from build123d import *

# Parameters (mm, degrees)
RESSALTO_EXTRUS_O1_DEPTH = 48
ESBO_O12_R               = 1.5
CORTE_EXTRUS_O10_DEPTH   = 10
ESBO_O13_R               = 1.5
CORTE_EXTRUS_O11_DEPTH   = 10
ESBO_O14_R               = 1.5
CORTE_EXTRUS_O12_DEPTH   = 10
ESBO_O15_R               = 1.5
CORTE_EXTRUS_O13_DEPTH   = 10
CORTE_EXTRUS_O14_DEPTH   = 10
CORTE_EXTRUS_O15_DEPTH   = 24
ESBO_O17_R               = 4
ESBO_O17_W               = 2.8
ESBO_O17_H               = 2.8
RESSALTO_EXTRUS_O2_DEPTH = 4
CORTE_EXTRUS_O16_DEPTH   = 24


with BuildPart() as part:
    # Model → Ressalto-extrusão1 (new body)
    with BuildSketch(Plane.XY):
        with BuildLine():
            Line((-0.7, 0), (39, 0))
            Line((39, 0), (39.7, 0))
            Line((39.7, 0), (39.7, -11.380317396))
            Line((39.7, -11.380317396), (50.182424304, -21.8627417))
            Line((50.182424304, -21.8627417), (58.119682605, -29.8))
            Line((58.119682605, -29.8), (81.7, -29.8))
            ThreePointArc((81.7, -29.8), (105.905643752, -13.626305928), (100.226197667, 14.926197667))
            Line((100.226197667, 14.926197667), (65.00338056, 50.149014774))
            Line((65.00338056, 50.149014774), (50.111140335, 50.149014774))
            Line((50.111140335, 50.149014774), (14.181595121, 50.149014774))
            Line((14.181595121, 50.149014774), (-3.2, 32.767419653))
            Line((-3.2, 32.767419653), (-3.2, 5))
            Line((-3.2, 5), (-3.2, 0))
            Line((-3.2, 0), (-0.7, 0))
        make_face()
        with BuildLine():
            Line((-0.7, 2.5), (39, 2.5))
            Line((39, 2.5), (39.7, 2.5))
            Line((39.7, 2.5), (42.2, 2.5))
            Line((42.2, 2.5), (42.2, -10.34478349))
            Line((42.2, -10.34478349), (51.950191257, -20.094974747))
            Line((51.950191257, -20.094974747), (59.15521651, -27.3))
            Line((59.15521651, -27.3), (81.7, -27.3))
            ThreePointArc((81.7, -27.3), (103.595944921, -12.669597347), (98.458430714, 13.158430714))
            Line((98.458430714, 13.158430714), (63.967846654, 47.649014774))
            Line((63.967846654, 47.649014774), (50.111140335, 47.649014774))
            Line((50.111140335, 47.649014774), (15.217129027, 47.649014774))
            Line((15.217129027, 47.649014774), (-0.7, 31.731885747))
            Line((-0.7, 31.731885747), (-0.7, 2.5))
        make_face(mode=Mode.SUBTRACT)
    extrude(amount=RESSALTO_EXTRUS_O1_DEPTH)

    # Esboço12 → Corte-extrusão10 (cut)
    with BuildSketch(Plane(origin=(57.576197667, 57.576197667, 0), x_dir=(0, 0, -1), z_dir=(0.707106781, 0.707106781, 0))):
        with Locations((-44, -20.072657306)):
            Circle(ESBO_O12_R)
        with Locations((-44, -52.072657306)):
            Circle(ESBO_O12_R)
    extrude(amount=-CORTE_EXTRUS_O10_DEPTH, mode=Mode.SUBTRACT)

    # Esboço13 → Corte-extrusão11 (cut)
    with BuildSketch(Plane(origin=(0, 50.149014774, 0), x_dir=(1, 0, 0), z_dir=(0, 1, 0))):
        with Locations((39.59248784, -44)):
            Circle(ESBO_O13_R)
    extrude(amount=-CORTE_EXTRUS_O11_DEPTH, mode=Mode.SUBTRACT)

    # Esboço14 → Corte-extrusão12 (cut)
    with BuildSketch(Plane.ZY.offset(3.2)):
        with Locations((44, 23.701037279)):
            Circle(ESBO_O14_R)
        with Locations((44, 7.740898975)):
            Circle(ESBO_O14_R)
    extrude(amount=-CORTE_EXTRUS_O12_DEPTH, mode=Mode.SUBTRACT)

    # Esboço15 → Corte-extrusão13 (cut)
    with BuildSketch(Plane(origin=(14.159841302, 14.159841302, 0), x_dir=(0, 0, 1), z_dir=(-0.707106781, -0.707106781, 0))):
        with Locations((44, -46.881179593)):
            Circle(ESBO_O15_R)
    extrude(amount=-CORTE_EXTRUS_O13_DEPTH, mode=Mode.SUBTRACT)

    # Esboço16 → Corte-extrusão14 (cut)
    with BuildSketch(Plane.XY.offset(48)):
        Polygon((39.7, 0), (39.7, -7.84478349), (42.2, -10.34478349), (42.2, 2.5), (-0.7, 2.5), (-0.7, 0), align=None)
    extrude(amount=-CORTE_EXTRUS_O14_DEPTH, mode=Mode.SUBTRACT)

    # Esboço18 → Corte-extrusão15 (cut)
    with BuildSketch(Plane(origin=(0, 0, 0), x_dir=(-1, 0, 0), z_dir=(0, 0, -1))):
        with BuildLine():
            Line((-39.7, 0), (3.2, 0))
            Line((3.2, 0), (3.2, 32.767419653))
            Line((3.2, 32.767419653), (-14.181595121, 50.149014774))
            Line((-14.181595121, 50.149014774), (-65.00338056, 50.149014774))
            Line((-65.00338056, 50.149014774), (-100.226197667, 14.926197667))
            ThreePointArc((-100.226197667, 14.926197667), (-105.905643752, -13.626305928), (-81.7, -29.8))
            Line((-81.7, -29.8), (-58.119682605, -29.8))
            Line((-58.119682605, -29.8), (-39.7, -11.380317396))
            Line((-39.7, -11.380317396), (-39.7, 0))
        make_face()
    extrude(amount=-CORTE_EXTRUS_O15_DEPTH, mode=Mode.SUBTRACT)

    # Esboço17 → Ressalto-extrusão2 (add)
    with BuildSketch(Plane(origin=(0, 0, 24), x_dir=(-1, 0, 0), z_dir=(0, 0, -1))):
        with Locations((-91.568699638, 17.926841447)):
            Circle(ESBO_O17_R)
        with Locations((-91.568699638, 17.926841447)):
            Rectangle(ESBO_O17_W, ESBO_O17_H, mode=Mode.SUBTRACT)
        with Locations((-68.47265349, 41.022887595)):
            Circle(ESBO_O17_R)
        with Locations((-68.47265349, 41.022887595)):
            Rectangle(ESBO_O17_W, ESBO_O17_H, mode=Mode.SUBTRACT)
        with Locations((-39.59248784, 46.149014774)):
            Circle(ESBO_O17_R)
        with Locations((-39.59248784, 46.149014774)):
            Rectangle(ESBO_O17_W, ESBO_O17_H, mode=Mode.SUBTRACT)
        with Locations((-0.8, 24.383709827)):
            Circle(ESBO_O17_R)
        with Locations((-0.8, 24.383709827)):
            Rectangle(ESBO_O17_W, ESBO_O17_H, mode=Mode.SUBTRACT)
        with Locations((-0.8, 8.383709827)):
            Circle(ESBO_O17_R)
        with Locations((-0.8, 8.383709827)):
            Rectangle(ESBO_O17_W, ESBO_O17_H, mode=Mode.SUBTRACT)
        with Locations((-51.388268427, -17.411731573)):
            Circle(ESBO_O17_R)
        with Locations((-51.388268427, -17.411731573)):
            Rectangle(ESBO_O17_W, ESBO_O17_H, mode=Mode.SUBTRACT)
    extrude(amount=-RESSALTO_EXTRUS_O2_DEPTH)


with BuildPart() as body_2:
    # Espelhar2: mirrored copy
    add(part.part.mirror(Plane(origin=(81.7, -3.6, 48), x_dir=(1, 0, 0), z_dir=(0, 0, 1))))


with BuildPart() as part_1:
    add(part.part)

    # Esboço19 → Corte-extrusão16 (cut)
    with BuildSketch(Plane(origin=(0, 0, 24), x_dir=(-1, 0, 0), z_dir=(0, 0, -1))):
        with BuildLine():
            Line((-58.119682605, -29.8), (-39.7, -11.380317396))
            Line((-39.7, -11.380317396), (-39.7, 0))
            Line((-39.7, 0), (3.2, 0))
            Line((3.2, 0), (3.2, 32.767419653))
            Line((3.2, 32.767419653), (-14.181595121, 50.149014774))
            Line((-14.181595121, 50.149014774), (-65.00338056, 50.149014774))
            Line((-65.00338056, 50.149014774), (-100.226197667, 14.926197667))
            ThreePointArc((-100.226197667, 14.926197667), (-105.905643752, -13.626305928), (-81.7, -29.8))
            Line((-81.7, -29.8), (-58.119682605, -29.8))
        make_face()
    extrude(amount=-CORTE_EXTRUS_O16_DEPTH, mode=Mode.SUBTRACT)


solid = body_2.part
Can you work these out from the model? Positions are in its coordinate system, mm. A direction names the side the tool comes from. Coordinates: 2 decimals unless noted, no trailing zeros. Write each loop counter-clockwise with the first axis right and the second up, starting at its lowest first coordinate (ties: lowest second). Pieces come first, ordered by that corner, then holes.
Q1. Imagine slicing it at D-D, the plane z = 52. Count the separate pieces of the cut face and the enclosed holes in it, plus the area to 3 significant figures.
Results found:
separate pieces: 7
enclosed holes: 0
area: 614 mm2
Q2. Imagine slicing it at A-A, the plane x = 25. List the corners of the cut face in (y, z) for me, plus the area to 3 significant figures.
Results found:
outline: (0, 58) - (2.5, 58) - (2.5, 72) - (0, 72) - close; (47.65, 48) - (50.15, 48) - (50.15, 72) - (47.65, 72) - close
area: 95.0 mm2
Q3. For P1, Ø12, axis at x = 13, z = 64, coming from the -Y side; P2, Ø3, axis at y = 9, z = 70.5, coming from the +X side; P3, Ø11.5, axis at x = 73.5, z = 54, coming from the +Y side, each with a flat end and sliding along its axis, tell me the tip position at first contact or that it passes through.
Results found:
P1: stops at y = 0
P2: stops at x = 105.43
P3: stops at y = 47.4
Q4. Which directions (+Z, -Z, +X, -X, +Y, -Y) give clear straight access to the entire face, cutting with the end or side of a thin tool? Please do faces 1 (the face through (49.988, -17, 70)), 2 (the face through (-1.97, 6.83, 53.19)), 3 (the face through (40, 44, 68)).
Results found:
face 1: +Z, -Z
face 2: -X
face 3: -Z
Q5. Imagine slicing it at B-B, the plane x = 0.8. List the corners of the cut face in (y, z) for me, plus the area to 3 significant figures.
Results found:
outline: (0, 58) - (2.5, 58) - (2.5, 72) - (0, 72) - close; (4.38, 68) - (6.98, 68) - (6.98, 72) - (4.38, 72) - close; (9.78, 68) - (12.38, 68) - (12.38, 72) - (9.78, 72) - close; (20.38, 68) - (22.98, 68) - (22.98, 72) - (20.38, 72) - close; (25.78, 68) - (28.38, 68) - (28.38, 72) - (25.78, 72) - close; (33.23, 48) - (36.77, 48) - (36.77, 72) - (33.23, 72) - close
area: 161 mm2
Q6. Imagine slicing it at C-C, the plane y = -3.5. List the corners of the cut face in (x, z) for me.
Results found:
outline: (39.7, 58) - (42.2, 58) - (42.2, 72) - (39.7, 72) - close; (105.4, 48) - (107.9, 48) - (107.9, 72) - (105.4, 72) - close
Q7. Please list where these lines run through material, in increasing order: L1, parallel to Y at x = 36.5, z = 63.5; L2, parallel to Y at x = -2.6, z = 52; L3, parallel to Y at x = 69, z = 69.25.
Results found:
L1: y = 0 to 2.5, 47.65 to 50.15
L2: y = 0 to 6.24, 9.24 to 22.2, 25.2 to 33.37
L3: y = -29.8 to -27.3, 37.06 to 39.62, 42.42 to 46.15
Q8. If we mould it in two halves opening along Y, with no side actions, what happens to faces 4 (the face through (-0.6, 24, 70)), 5 (the face through (40, 1, 72))? For each: +Y half, -Y half, draft (parallel to the pull), parting line (faces both ways), or undercut.
Results found:
face 4: undercut
face 5: draft
